Can you work these out from the model? Positions are in its coordinate system, mm. A direction names the side the tool comes from. Give positions to 0.01 mm unless a question says otherwise; leave off trailing zeros. Loops run counter-clockwise (first coordinate to the right, second up) from the corner with the lowest first, then second, coordinate; pieces in that order, holes last. Notation, with made-up numbers: (25.25, -15) -> (64.25, -15) arc R23 ccw to (64.25, 7) -> close; hole circle Ø5 at (44, -37.75). An arc over 180 degrees is marked (long way). Return JSON: item names as keys, results as strings. Group by question number.
Q1. Thinking about a two-plate mould opening in Y: for faces 1 (the cylindrical face through (37.651, 11.132, 13.804)), 2 (the flat face through (0, 37, 11)), 3 (the cylindrical face through (21.723, 17.802, 30.958)), 4 (the flat face through (40, 38, 10)), which applies, pulls with the +Y half, pulls with the -Y half, needs draft (parallel to the pull), parting line crosses it, or undercut?
Q2. Will these pins go through, and if not, where does the flat tip stop? pin 1 (9.5 mm diameter, centred on x = 25.5, z = 10, fed in from +Y); pin 2 (6 mm diameter, centred on x = 49, y = 12, fed in from +Z); pin 3 (2.5 mm diameter, centred on y = 32, z = 14, fed in from +X).
Q3. I need wall thicknesses on line 1 along Y through (x, z) = (44, 22.5); line 2 along Y through (x, z) = (44, 6); line 3 along Z through (x, y) = (15.5, 37). Which ranges of each line are inside material? Lowest first, please. Write a range as [from, to].
Q4. Suppose I cut it at C-C, the plane z = 17. Please give me the cut outline in (x, y), and give its area (3 significant figures).
Q5. Suppose I cut it at D-D, the plane x = 16. Please give me the cut outline in (y, z), and give its area (3 significant figures).
Q6. Which directions (+Z, -Z, +X, -X, +Y, -Y) give clear straight access to the entire face, cutting with the end or side of a thin tool? Please do faces 5 (the flat face through (48, 34, 10)), 6 (the flat face through (60, 15, 14)), 7 (the flat face through (19, 48, 20)).
Q7. Suppose I cut it at A-A, the plane x = 44. Please give me the cut outline in (y, z), and give its area (3 significant figures).
Q8. Suppose I cut it at B-B, the plane y = 16. Please give me the cut outline in (x, z), and give its area (3 significant figures).
```python
from build123d import *

# Parameters (mm, degrees)
SKETCH1_W           = 60
SKETCH1_H           = 30
SKETCH1_R           = 8
BOSS_EXTRUDE1_DEPTH = 28
BOSS_EXTRUDE2_DEPTH = 20
SKETCH3_R           = 6
BOSS_EXTRUDE3_DEPTH = 6


with BuildPart() as part:
    # Sketch1 → Boss-Extrude1 (new body)
    with BuildSketch(Plane.XY):
        with Locations((30, 15)):
            Rectangle(SKETCH1_W, SKETCH1_H)
        with Locations((44, 16)):
            Circle(SKETCH1_R, mode=Mode.SUBTRACT)
    extrude(amount=BOSS_EXTRUDE1_DEPTH)

    # Sketch2 → Boss-Extrude2 (add)
    with BuildSketch(Plane.XY):
        Polygon((0, 30), (0, 75), (20, 75), (20, 50), (32, 50), (32, 38), (48, 38), (48, 30), align=None)
    extrude(amount=BOSS_EXTRUDE2_DEPTH)

    # Sketch3 → Boss-Extrude3 (add)
    with BuildSketch(Plane.XY.offset(28)):
        with Locations((16, 16)):
            Circle(SKETCH3_R)
    extrude(amount=BOSS_EXTRUDE3_DEPTH)


solid = part.part
```
Ans:
{
 "1": {"face 1": "undercut", "face 2": "needs draft", "face 3": "parting line crosses it", "face 4": "pulls with the +Y half"},
 "2": {"pin 1": "stops at y = 50", "pin 2": "stops at z = 28", "pin 3": "stops at x = 48"},
 "3": {"line 1": "y = [0, 8], [24, 30]", "line 2": "y = [0, 8], [24, 38]", "line 3": "z = [0, 20]"},
 "4": {"outline": "(0, 0) -> (60, 0) -> (60, 30) -> (48, 30) -> (48, 38) -> (32, 38) -> (32, 50) -> (20, 50) -> (20, 75) -> (0, 75) -> close; hole circle Ø16 at (44, 16)", "area": "2,870 mm^2"},
 "5": {"outline": "(0, 0) -> (75, 0) -> (75, 20) -> (30, 20) -> (30, 28) -> (22, 28) -> (22, 34) -> (10, 34) -> (10, 28) -> (0, 28) -> close", "area": "1,810 mm^2"},
 "6": {"face 5": "+Z, -Z, +X, +Y", "face 6": "+Z, -Z, +X, +Y, -Y", "face 7": "+Z, +X, -X, +Y"},
 "7": {"outline": "(0, 0) -> (8, 0) -> (8, 28) -> (0, 28) -> close; (24, 0) -> (38, 0) -> (38, 20) -> (30, 20) -> (30, 28) -> (24, 28) -> close", "area": "552 mm^2"},
 "8": {"outline": "(0, 0) -> (36, 0) -> (36, 28) -> (22, 28) -> (22, 34) -> (10, 34) -> (10, 28) -> (0, 28) -> close; (52, 0) -> (60, 0) -> (60, 28) -> (52, 28) -> close", "area": "1,300 mm^2"}
}
